Autodesk Inventor part; units mm, degrees
ref_plane "YZ Plane" through (0, 0, 0) normal (1, 0, 0) x (0, 1, 0)
ref_plane "XZ Plane" through (0, 0, 0) normal (0, 1, 0) x (-1, 0, 0)
ref_plane "XY Plane" through (0, 0, 0) normal (0, 0, 1) x (1, 0, 0)
sketch "Sketch1" plane through (0, 0, 0) normal (0, 1, 0) x (-1, 0, 0)
  circle A0 centre (0, 0) radius 3.2339
extrude "Extrusion1" add sketch "Sketch1" along normal blind 2
sketch "Sketch2" plane through (0, 2, 0) normal (0, 1, 0) x (1, 0, 0)
  circle A0 centre (0, 0) radius 2.2475
extrude "Extrusion2" add sketch "Sketch2" along normal blind 1.5
fillet "Fillet1" radius 1.4 1 edges at (-2.2475, 2, 0)
sketch "Sketch3" plane through (0, 3.5, 0) normal (0, 1, 0) x (1, 0, 0)
  circle A0 centre (0, 0) radius 1.5857
extrude "Extrusion3" add sketch "Sketch3" along normal blind 0.5
sketch "Sketch4" plane through (0, 4, 0) normal (0, 1, 0) x (1, 0, 0)
  point P0 (0, 0)
properties part number "SWITCH"
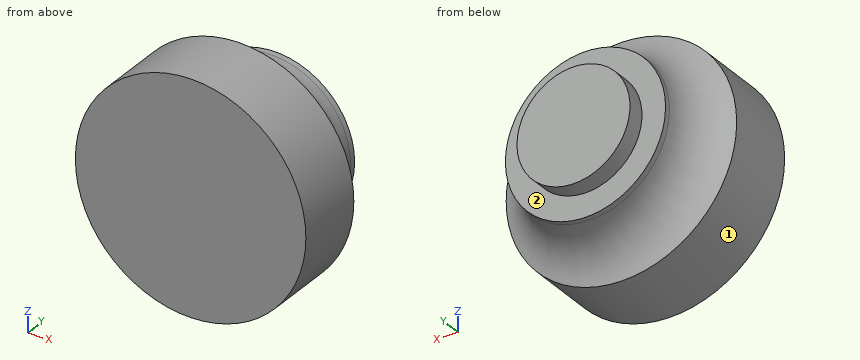
Model file for the job. Use its own axes, mm. Face numbers are marked on the shaded views. A direction names the side the tool comes from. Round coordinates to 2 decimals unless told otherwise and drop trailing zeros. Order: outer loops, then holes, each group sorted by start corner. A loop starts at its lowest first (then second) coordinate and runs counter-clockwise, first axis right, second up. Notation, with made-up numbers: M -37,-37.5 L 15,-37.5 A26 ccw 15,-13.5 Z; hole C 62.25,74 d6. An arc over 180 degrees is marked long. Use CSV: the item, a comma, the result in double quotes.
Item 1: Saw through at A-A (x = 0). List the corners of the cut face in (y, z).
Worked answers:
outline,"M 0,-3.23 L 2,-3.23 A1.4 cw 3.34,-2.25 L 3.5,-2.25 L 3.5,-1.59 L 4,-1.59 L 4,1.59 L 3.5,1.59 L 3.5,2.25 L 3.34,2.25 A1.4 cw 2,3.23 L 0,3.23 Z"
Item 2: Probe probe 1 along Y at (x, z) = (2.5, -0.75); probe 2 along X at (y, z) = (1, -2.5); probe 3 along X at (y, z) = (2.8, 2). List the from-to ranges inside material, lowest first.
Worked answers:
probe 1,"0 to 2.4"
probe 2,"-2.05 to 2.05"
probe 3,"-1.24 to 1.24"
Item 3: Pin check, flat tips, straight feed: pin 1 (1 mm diameter, centred on x = -2, z = -1.5, fed in from +Y); pin 2 (2 mm diameter, centred on y = 2, z = 2, fed in from -X). Stop position of each tip, or through.
Worked answers:
pin 1,"y = 3.5"
pin 2,"x = -3.08"
Item 4: Saw through at B-B (z = 0). List the corners of the cut face in (x, y), plus the area to 3 significant figures.
Worked answers:
outline,"M -3.23,0 L 3.23,0 L 3.23,2 A1.4 cw 2.25,3.34 L 2.25,3.5 L 1.59,3.5 L 1.59,4 L -1.59,4 L -1.59,3.5 L -2.25,3.5 L -2.25,3.34 A1.4 cw -3.23,2 Z"
area,"22.0 mm²"
Item 5: Which spindle directions (+Z, -Z, +X, -X, +Y, -Y) get a long thin tool onto all of the face, cutting with end or side? Do the marked faces 1 and 2. Say none if no direction does.
Worked answers:
face 1,"+Y, -Y"
face 2,"+Y"
